```python
from build123d import *

# Parameters (mm, degrees)
F1_DEPTH = 20
F0_R     = 3
F0_R_2   = 1.1
F2_DEPTH = 2
F3_DEPTH = 10.75
F0_W     = 3.1642657705
F0_H     = 1.4890261218
F4_DEPTH = 7
F5_R     = 2


# Not quite as in the source:
# - a feature names something its author has since deleted; it is built from what else it names


with BuildPart() as f1:
    # F0 (on Top) → F1 (new body)
    with BuildSketch(Plane.XY):
        Polygon((-37.55, -13.0740804598), (-37.55, -12.1), (-37.55, 13.5259195402), (37.55, 13.5259195402), (37.55, 2.0000108369), (39.55, 2.0000108369), (39.55, 15.7519578086), (-39.5226512551, 15.7519578086), (-39.5226512551, -46.2480421914), (39.55, -46.2480421914), (39.55, -1.9999891631), (37.55, -1.9999891631), (37.55, -13.0740804598), (-4.9305087887, -13.0740804598), (-4.9305087887, -14.5631065816), (36.1, -14.5631065816), (37.55, -14.5631065816), (37.55, -44.3981406778), (-37.55, -44.3981406778), (-37.55, -14.5631065816), (-36.1, -14.5631065816), (-8.0947745591, -14.5631065816), (-8.0947745591, -13.0740804598), align=None)
    extrude(amount=F1_DEPTH)



with BuildPart() as f1b:
    # F0 (on Top) → F1, piece 2 (new body)
    with BuildSketch(Plane.XY):
        with Locations((-30.2370786667, -18.2506926358)):
            Circle(F0_R)
        with Locations((-30.2370786667, -18.2506926358)):
            Circle(F0_R_2, mode=Mode.SUBTRACT)
    extrude(amount=F1_DEPTH)


with BuildPart() as f1c:
    # F0 (on Top) → F1, piece 3 (new body)
    with BuildSketch(Plane.XY):
        with Locations((30.2370786667, -18.2506926358)):
            Circle(F0_R)
        with Locations((30.2370786667, -18.2506926358)):
            Circle(F0_R_2, mode=Mode.SUBTRACT)
    extrude(amount=F1_DEPTH)


with BuildPart() as f2:
    # F0 (on Top) → F2 (new body)
    with BuildSketch(Plane.XY):
        with BuildLine():
            Line((-25.6, 1.6), (-25.6, 2.7))
            ThreePointArc((-25.6, 2.7), (-26.3778174593, 0.8221825407), (-24.5, 1.6))
            Line((-24.5, 1.6), (-25.6, 1.6))
        make_face()
        with BuildLine():
            ThreePointArc((-24.5, 1.6), (-24.8221825407, 2.3778174593), (-25.6, 2.7))
            Line((-25.6, 2.7), (-25.6, 1.6))
            Line((-25.6, 1.6), (-24.5, 1.6))
        make_face()
    extrude(amount=F2_DEPTH)


with BuildPart() as f2b:
    # F0 (on Top) → F2, piece 2 (new body)
    with BuildSketch(Plane.XY):
        with BuildLine():
            ThreePointArc((30.2, 2.1), (29.8778174593, 2.8778174593), (29.1, 3.2))
            ThreePointArc((29.1, 3.2), (28.3221825407, 1.3221825407), (30.2, 2.1))
        make_face()
    extrude(amount=F2_DEPTH)


with BuildPart() as f1_1:
    add(f1.part)

    add(f1b.part)  # F2#3 merges F1b

    add(f1c.part)  # F2#3 merges F1c
    # F0 (on Top) → F2, piece 3 (join)
    with BuildSketch(Plane.XY):
        Polygon((-4.9305087887, -14.5631065816), (-8.0947745591, -14.5631065816), (-36.1, -14.5631065816), (-36.1, -42.9981406778), (36.1, -42.9981406778), (36.1, -14.5631065816), align=None)
        with Locations((-30.2370786667, -18.2506926358)):
            Circle(F0_R, mode=Mode.SUBTRACT)
        with Locations((30.2370786667, -18.2506926358)):
            Circle(F0_R, mode=Mode.SUBTRACT)
        Polygon((-37.55, 13.5259195402), (-37.55, -12.1), (-37.55, -13.0740804598), (-8.0947745591, -13.0740804598), (-4.9305087887, -13.0740804598), (37.55, -13.0740804598), (37.55, -1.9999891631), (37.55, 2.0000108369), (37.55, 13.5259195402), align=None)
        Polygon((36.1, 12.1), (36.1, -12.1), (-36.1, -12.1), (-36.1, 12.1), (-25.6, 12.1), (29.1, 12.1), align=None, mode=Mode.SUBTRACT)
        Polygon((-36.1, -12.1), (36.1, -12.1), (36.1, 12.1), (29.1, 12.1), (-25.6, 12.1), (-36.1, 12.1), align=None)
        with BuildLine():
            ThreePointArc((-22.6, 1.6), (-27.7213203436, -0.5213203436), (-25.6, 4.6))
            ThreePointArc((-25.6, 4.6), (-23.4786796564, 3.7213203436), (-22.6, 1.6))
        make_face(mode=Mode.SUBTRACT)
        with BuildLine():
            ThreePointArc((32.1000297599, 2.1), (26.978658613, -0.021341387), (29.1, 5.1000297599))
            ThreePointArc((29.1, 5.1000297599), (31.221341387, 4.221341387), (32.1000297599, 2.1))
        make_face(mode=Mode.SUBTRACT)
        Polygon((-36.1, -42.9981406778), (-36.1, -14.5631065816), (-37.55, -14.5631065816), (-37.55, -44.3981406778), (37.55, -44.3981406778), (37.55, -14.5631065816), (36.1, -14.5631065816), (36.1, -42.9981406778), align=None)
        with Locations((-30.2370786667, -18.2506926358)):
            Circle(F0_R_2)
        with Locations((30.2370786667, -18.2506926358)):
            Circle(F0_R_2)
    extrude(amount=F2_DEPTH)


    add(f2.part)  # F3 merges F2

    add(f2b.part)  # F3 merges F2b
    # F0 (on Top) → F3 (join)
    with BuildSketch(Plane.XY):
        with BuildLine():
            Line((-25.6, 2.7), (-25.6, 4.6))
            ThreePointArc((-25.6, 4.6), (-27.7213203436, -0.5213203436), (-22.6, 1.6))
            Line((-22.6, 1.6), (-24.5, 1.6))
            ThreePointArc((-24.5, 1.6), (-26.3778174593, 0.8221825407), (-25.6, 2.7))
        make_face()
        with BuildLine():
            ThreePointArc((-22.6, 1.6), (-23.4786796564, 3.7213203436), (-25.6, 4.6))
            Line((-25.6, 4.6), (-25.6, 2.7))
            ThreePointArc((-25.6, 2.7), (-24.8221825407, 2.3778174593), (-24.5, 1.6))
            Line((-24.5, 1.6), (-22.6, 1.6))
        make_face()
        with BuildLine():
            ThreePointArc((32.1000297599, 2.1), (31.221341387, 4.221341387), (29.1, 5.1000297599))
            ThreePointArc((29.1, 5.1000297599), (26.978658613, -0.021341387), (32.1000297599, 2.1))
        make_face()
        with BuildLine():
            ThreePointArc((30.2, 2.1), (28.3221825407, 1.3221825407), (29.1, 3.2))
            ThreePointArc((29.1, 3.2), (29.8778174593, 2.8778174593), (30.2, 2.1))
        make_face(mode=Mode.SUBTRACT)
    extrude(amount=F3_DEPTH)

    # F0 (on Top) → F4 (join)
    with BuildSketch(Plane.XY):
        Polygon((39.55, 2.0000108369), (37.55, 2.0000108369), (37.55, -1.9999891631), (39.55, -1.9999891631), (39.55, 1.08369e-05), align=None)
        with Locations((-6.5126416739, -13.8185935207)):
            Rectangle(F0_W, F0_H)
    extrude(amount=F4_DEPTH)

    # F5
    f5_edges = [f1_1.edges().sort_by_distance(p)[0] for p in [
        (39.55, -46.248042, 10),
        (39.55, 15.751958, 10),
        (-39.522651, 15.751958, 10),
        (-39.522651, -46.248042, 10),
    ]]
    fillet(f5_edges, radius=F5_R)


solid = f1_1.part
```
Geometry: final body of the model. Coordinates: model frame, mm. A direction names the side the tool comes from. Coordinates: 2 decimals unless noted, no trailing zeros. Order: outer loops, then holes, each group sorted by start corner. A loop starts at its lowest first (then second) coordinate and runs counter-clockwise, first axis right, second up. Notation, with made-up numbers: M 22.25,74.5 L 63.25,74.5 A19 ccw 63.25,89.5 Z; hole C 83,17 d4. An arc over 180 degrees is marked long. Answer in a Markdown table with one row per item. Add a question column.
Q1. Mould query, pull axis Y, two halves, no side actions, for faces 1 (the cylindrical face through (-27.466, -19.4, 10.874)), 2 (the cylindrical face through (-38.9, 15.2, 10.1)), 3 (the flat face through (39.55, -16, 10)). Classes: released by +Y, released by -Y, zero draft, split by the parting line, or undercut.
Q2. Section query C-C on y = -42. Return the cut outline in (x, z), and give its area (3 significant figures).
Q3. Section query B-B on x = -18. Return the cut outline in (y, z), and give its area (3 significant figures).
Q4. Section query D-D on z = 16. Return the cut outline in (x, y).
Q5. Section query A-A on z = 4. Count the separate pieces of the cut face and the enclosed holes in it, and give its area (3 significant figures).
Q6. Line query: L1, parallel to Y at x = -0.5, z = 17.25; L2, parallel to X at y = -6, z = 16.75; L3, parallel to Y at x = -32, z = 6.25. Output: solid intervals per line, ascending.
Q7. Reachability of faces 4 (the flat face through (39, 2, 13)), 5 (the cylindrical face through (38.98, -45.647, 10.14)), 6 (the flat face through (-1, 13.526, 11)) from +Z, -Z, +X, -X, +Y, -Y: full face, straight path, thin tool, end or side. Return the list, or none.
Q8. Contact query for flat-ended pins moving along their axis: P1, Ø0.6, axis at x = 38.5, y = 1, coming from the +Z side; P2, Ø2.5, axis at x = -26, y = 2, coming from the +Z side; P3, Ø8, axis at x = 14.5, y = 6.5, coming from the +Z side. Output: stop coordinate, or through.
Completed:
| question | item | result |
|---|---|---|
| 1 | face 1 | undercut |
| 1 | face 2 | released by +Y |
| 1 | face 3 | zero draft |
| 2 | outline | M -39.52,0 L 39.55,0 L 39.55,20 L 37.55,20 L 37.55,2 L -37.55,2 L -37.55,20 L -39.52,20 Z |
| 2 | area | 230 mm2 |
| 3 | outline | M -46.25,0 L 15.75,0 L 15.75,20 L 13.53,20 L 13.53,2 L -13.07,2 L -13.07,20 L -14.56,20 L -14.56,2 L -44.4,2 L -44.4,20 L -46.25,20 Z |
| 3 | area | 224 mm2 |
| 4 | outline | M -39.52,-44.25 A2 ccw -37.52,-46.25 L 37.55,-46.25 A2 ccw 39.55,-44.25 L 39.55,-2 L 37.55,-2 L 37.55,-13.07 L -4.93,-13.07 L -4.93,-14.56 L 37.55,-14.56 L 37.55,-44.4 L -37.55,-44.4 L -37.55,-14.56 L -8.09,-14.56 L -8.09,-13.07 L -37.55,-13.07 L -37.55,13.53 L 37.55,13.53 L 37.55,2 L 39.55,2 L 39.55,13.75 A2 ccw 37.55,15.75 L -37.52,15.75 A2 ccw -39.52,13.75 Z; C -30.24,-18.25 d6; C 30.24,-18.25 d6; hole C -30.24,-18.25 d2.2; hole C 30.24,-18.25 d2.2 |
| 5 | separate pieces | 5 |
| 5 | enclosed holes | 6 |
| 5 | area | 759 mm2 |
| 6 | L1 | y = -46.25 to -44.4, -14.56 to -13.07, 13.53 to 15.75 |
| 6 | L2 | x = -39.52 to -37.55, 37.55 to 39.55 |
| 6 | L3 | y = -46.25 to -44.4, -20.68 to -15.82, -14.56 to -13.07, 13.53 to 15.75 |
| 7 | face 4 | +Z, +X |
| 7 | face 5 | +Z, -Z, +X, -Y |
| 7 | face 6 | +Z |
| 8 | P1 | stops at z = 7 |
| 8 | P2 | stops at z = 10.75 |
| 8 | P3 | stops at z = 2 |
